```python
from build123d import *

# Parameters (mm, degrees)
BODY_DEPTH            = 3.175
FILLET1_R             = 6.35
F_6_32_TAPPED_HOLE1_D = 2.7051
F_6_CLEARANCE_HOLE2_D = 3.7973


with BuildPart() as part:
    # Sketch1 → Body (new body)
    with BuildSketch(Plane.XY):
        with BuildLine():
            Line((-6.35, 100.140279829), (-29.36875, 100.140279829))
            Line((-29.36875, 100.140279829), (-29.36875, 87.633226142))
            Line((-29.36875, 87.633226142), (29.36875, 87.633226142))
            Line((29.36875, 87.633226142), (29.36875, 100.140279829))
            Line((29.36875, 100.140279829), (6.35, 100.140279829))
            Line((6.35, 100.140279829), (6.35, 117.602779829))
            ThreePointArc((6.35, 117.602779829), (0, 123.952779829), (-6.35, 117.602779829))
            Line((-6.35, 117.602779829), (-6.35, 100.140279829))
        make_face()
    extrude(amount=BODY_DEPTH)

    # Fillet1
    # the kernel refuses this fillet: 6.35 mm, written as the material it adds along each edge
    with BuildSketch(Plane(origin=(6.35, 100.140279829, 0), x_dir=(1, 0, 0), z_dir=(0, 0, 1)), Plane(origin=(-6.35, 100.140279829, 0), x_dir=(0, 1, 0), z_dir=(0, 0, 1))) as fillet1_piece_1:
        with BuildLine():
            CenterArc((FILLET1_R, FILLET1_R), FILLET1_R, 180, 90)
            Line((0, FILLET1_R), (0, 0))
            Line((0, 0), (FILLET1_R, 0))
        make_face()
    extrude(amount=3.175)
    # the kernel refuses this fillet: 6.35 mm, written as the material it takes off along each edge
    with BuildSketch(Plane(origin=(29.36875, 87.633226142, -15.875), x_dir=(-1, 0, 0), z_dir=(0, 0, 1)), Plane(origin=(29.36875, 100.140279829, -15.875), x_dir=(0, -1, 0), z_dir=(0, 0, 1)), Plane(origin=(-29.36875, 100.140279829, -15.875), x_dir=(1, 0, 0), z_dir=(0, 0, 1)), Plane(origin=(-29.36875, 87.633226142, -15.875), x_dir=(0, 1, 0), z_dir=(0, 0, 1))) as fillet1_2_piece_1:
        with BuildLine():
            CenterArc((FILLET1_R, -FILLET1_R), FILLET1_R, 90, 90)
            Line((0, -FILLET1_R), (0, 0))
            Line((0, 0), (FILLET1_R, 0))
        make_face()
    extrude(amount=34.925, mode=Mode.SUBTRACT)

    # #6-32 Tapped Hole1 (through all)
    with Locations(Plane(origin=(20.32, 93.790279829, 0), x_dir=(-1, 0, 0), z_dir=(0, 0, -1))):
        with Locations((0, 0), (20.32, 0), (40.64, 0)):
            Hole(F_6_32_TAPPED_HOLE1_D / 2)

    # #6 Clearance Hole2 (through all)
    with Locations(Plane(origin=(0, 119.190279829, 0), x_dir=(-1, 0, 0), z_dir=(0, 0, -1))):
        with Locations((0, 0), (-25.4316925, 83.647585323), (0, -11.1125)):
            Hole(F_6_CLEARANCE_HOLE2_D / 2)


solid = part.part
```
Source: CAD feature listing. Evaluate the final solid. Frame: model axes, mm. A direction names the side the tool comes from. Round coordinates to 2 decimals unless told otherwise and drop trailing zeros. Loops run counter-clockwise (first coordinate to the right, second up) from the corner with the lowest first, then second, coordinate; pieces in that order, holes last.
1. Section query D-D on z = 0.55. Output: boundary loops of the cut face in (x, y), and give its area (3 significant figures).
2. Contact query for flat-ended pins moving along their axis: pin 1 (2 mm diameter, centred on x = 20.32, y = 93.79, fed in from +Z); pin 2 (1.6 mm diameter, centred on y = 111.5, z = 1.5, fed in from -X); pin 3 (1.6 mm diameter, centred on x = -17, z = 1, fed in from +Y). Output: stop coordinate, or through.
3. Access query for faces 4 (the cylindrical face through (27.425, 89.411, 1.565)), 5 (the flat face through (-6.35, 112, 2)), 6 (the flat face through (18, 100.14, 2)). Directions: +Z, -Z, +X, -X, +Y, -Y. A direction counts if a zero-diameter tool reaches every point of the face in a straight line with its end or side. Return the directions, or none.
4. Section query C-C on y = 120. Output: boundary loops of the cut face in (x, z) (3 decimals).
5. Section query A-A on x = 0. Output: boundary loops of the cut face in (y, z) (3 decimals).
6. Ray query, L1, parallel to Y at x = 0, z = 1.75; L2, parallel to X at y = 95, z = 1.75; L3, parallel to X at y = 107, z = 2.25. Return the intervals inside material, ascending.
7. Mould query, pull axis X, two halves, no side actions, for faces 1 (the flat face through (6.35, 112, 2)), 2 (the cylindrical face through (1.02, 120.79, 1.61)), 3 (the flat face through (-18, 100.14, 2)). Classes: released by +X, released by -X, zero draft, split by the parting line, or undercut.
8. Section query B-B on x = -20.32. Output: boundary loops of the cut face in (y, z) (3 decimals).
Answers below:
1. outline: (-29.37, 93.89) arc R6.35 ccw to (-23.02, 87.63) - (23.02, 87.63) arc R6.35 ccw to (29.37, 93.89) arc R6.35 ccw to (23.02, 100.14) - (12.7, 100.14) arc R6.35 cw to (6.35, 106.49) - (6.35, 117.6) arc R6.35 ccw to (-6.35, 117.6) - (-6.35, 106.49) arc R6.35 cw to (-12.7, 100.14) - (-23.02, 100.14) arc R6.35 ccw to start; hole circle Ø2.71 at (-20.32, 93.79); hole circle Ø3.8 at (0, 108.08); hole circle Ø3.8 at (0, 119.19); hole circle Ø2.71 at (0, 93.79); hole circle Ø2.71 at (20.32, 93.79)
1. area: 963 mm2
2. pin 1: passes through
2. pin 2: stops at x = -6.35
2. pin 3: stops at y = 100.14
3. face 4: +Z, -Z, +X, -Y
3. face 5: +Z, -Z, -X, +Y
3. face 6: +Z, -Z, +X, +Y
4. outline: (-5.88, 0) - (-1.717, 0) - (-1.717, 3.175) - (-5.88, 3.175) - close; (1.717, 0) - (5.88, 0) - (5.88, 3.175) - (1.717, 3.175) - close
5. outline: (87.633, 0) - (92.438, 0) - (92.438, 3.175) - (87.633, 3.175) - close; (95.143, 0) - (106.179, 0) - (106.179, 3.175) - (95.143, 3.175) - close; (109.976, 0) - (117.292, 0) - (117.292, 3.175) - (109.976, 3.175) - close; (121.089, 0) - (123.953, 0) - (123.953, 3.175) - (121.089, 3.175) - close
6. L1: y = 87.63 to 92.44, 95.14 to 106.18, 109.98 to 117.29, 121.09 to 123.95
6. L2: x = -29.25 to -20.92, -19.72 to -0.6, 0.6 to 19.72, 20.92 to 29.25
6. L3: x = -6.35 to -1.56, 1.56 to 6.35
7. face 1: released by +X
7. face 2: undercut
7. face 3: zero draft
8. outline: (87.633, 0) - (92.438, 0) - (92.438, 3.175) - (87.633, 3.175) - close; (95.143, 0) - (100.14, 0) - (100.14, 3.175) - (95.143, 3.175) - close
